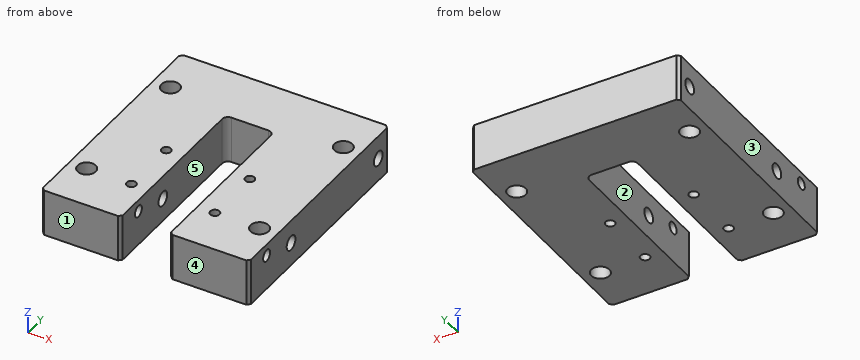
```python
from build123d import *

# Parameters (mm, degrees)
SKETCH_1_W          = 35.6
SKETCH_1_H          = 40
EXTRUDE_1_DEPTH     = 8
SKETCH_5_R          = 1
CUT_EXTRUDE_1_DEPTH = 42
SKETCH_6_W          = 8.3
SKETCH_6_H          = 60
CUT_EXTRUDE_2_DEPTH = 10
SKETCH_2_R          = 1.55
CUT_EXTRUDE_3_DEPTH = 10
HOLE_WIZARD_M2_1_D  = 1.6
HOLE_WIZARD_M3_2_D  = 2.5
FILLET_1_R          = 1
CHAMFER_1_SIZE      = 0.5


with BuildPart() as part:
    # 草图1 → 凸台-拉伸1 (new body)
    with BuildSketch(Plane.XY):
        Rectangle(SKETCH_1_W, SKETCH_1_H)
    extrude(amount=EXTRUDE_1_DEPTH)

    # 草图5 → 切除-拉伸1 (cut)
    with BuildSketch(Plane.ZY.offset(17.8)):
        with Locations((6, -15)):
            Circle(SKETCH_5_R)
    extrude(amount=-CUT_EXTRUDE_1_DEPTH, mode=Mode.SUBTRACT)

    # 草图6 → 切除-拉伸2 (cut)
    with BuildSketch(Plane.XY.offset(8)):
        with Locations((0, -20)):
            Rectangle(SKETCH_6_W, SKETCH_6_H)
    extrude(amount=-CUT_EXTRUDE_2_DEPTH, mode=Mode.SUBTRACT)

    # 草图2 → 切除-拉伸3 (cut)
    with BuildSketch(Plane.XY.offset(8)):
        with Locations((14.8, 12)):
            Circle(SKETCH_2_R)
        with Locations((-14.8, 12)):
            Circle(SKETCH_2_R)
        with Locations((-14.8, -12)):
            Circle(SKETCH_2_R)
        with Locations((14.8, -12)):
            Circle(SKETCH_2_R)
    extrude(amount=-CUT_EXTRUDE_3_DEPTH, mode=Mode.SUBTRACT)

    # M2 螺纹孔1 (through all)
    with Locations(Plane.XY.offset(8)):
        with Locations((-7.15, -12), (-7.15, -2)):
            hole_wizard_m2_1 = Hole(HOLE_WIZARD_M2_1_D / 2)

    # 镜向1: M2 螺纹孔1 across plane
    add(hole_wizard_m2_1.mirror(Plane(origin=(0, 0, 0), x_dir=(0, 0, 1), z_dir=(1, 0, 0))), mode=Mode.SUBTRACT)

    # M3 螺纹孔2 (through all)
    with Locations(Plane.ZY.offset(17.8)):
        with Locations((4, 17), (4, -8)):
            Hole(HOLE_WIZARD_M3_2_D / 2)

    # 圆角1
    fillet_1_edges = [part.edges().sort_by_distance(p)[0] for p in [
        (4.15, 10, 4),
        (-4.15, 10, 4),
    ]]
    fillet(fillet_1_edges, radius=FILLET_1_R)

    # 倒角1
    chamfer_1_edges = [part.edges().sort_by_distance(p)[0] for p in [
        (4.15, -20, 4),
        (-4.15, -20, 4),
        (17.8, -20, 4),
        (-17.8, -20, 4),
        (-17.8, 20, 4),
        (17.8, 20, 4),
    ]]
    chamfer(chamfer_1_edges, length=CHAMFER_1_SIZE)


solid = part.part
```
Model file for the job. Use its own axes, mm. Face numbers are marked on the shaded views. A direction names the side the tool comes from. Coordinates: 2 decimals unless noted, no trailing zeros. Order: outer loops, then holes, each group sorted by start corner. A loop starts at its lowest first (then second) coordinate and runs counter-clockwise, first axis right, second up. Notation, with made-up numbers: (66.5, 62.5) -> (110.5, 62.5) arc R20 ccw to (110.5, 98.5) -> close; hole circle Ø10 at (-7.75, -20). An arc over 180 degrees is marked (long way). Return JSON: item names as keys, results as strings.
Item 1: 3-axis set-ups, long thin cutter, end or side, ignore diameter. For the marked faces 1 and 2: which of +Z, -Z, +X, -X, +Y, -Y reach the whole face in a straight line?
Model answer:
{"face 1": "+Z, -Z, +X, -X, -Y", "face 2": "+Z, -Z, -Y"}
Item 2: Wall check: line 1 along Y through (x, z) = (9.25, 4); line 2 along Y through (x, z) = (7.15, 6); line 3 along Y through (x, z) = (11.5, 6). Give the ranges that are in metal, low to high. Write a range as from..to.
Model answer:
{"line 1": "y = -20..-9.25, -6.75..15.75, 18.25..20", "line 2": "y = -20..-16, -14..-12.8, -11.2..-2.8, -1.2..20", "line 3": "y = -20..-16, -14..20"}
Item 3: Slice it at C-C (y = 8). Write the cut outline in (x, z), then the cut area to 3 significant figures.
Model answer:
{"outline": "(-17.8, 0) -> (-4.15, 0) -> (-4.15, 8) -> (-17.8, 8) -> close; (4.15, 0) -> (17.8, 0) -> (17.8, 8) -> (4.15, 8) -> close", "area": "218 mm²"}
Item 4: Pin check, flat tips, straight feed: P1, Ø1.2, axis at y = -15, z = 6, coming from the -X side; P2, Ø4, axis at x = -0.5, z = 6, coming from the -Y side. Stop position of each tip, or through.
Model answer:
{"P1": "passes through", "P2": "stops at y = 10"}
Item 5: Slice it at B-B (z = 6). Count the separate pieces of the cut face and the enclosed holes in it, then the cut area to 3 significant figures.
Model answer:
{"separate pieces": "3", "enclosed holes": "8", "area": "1,080 mm²"}
Item 6: Slice it at A-A (x = 7.15). Write the cut outline in (y, z), then the cut area to 3 significant figures.
Model answer:
{"outline": "(-20, 0) -> (-12.8, 0) -> (-12.8, 8) -> (-20, 8) -> close; (-11.2, 0) -> (-2.8, 0) -> (-2.8, 8) -> (-11.2, 8) -> close; (-1.2, 0) -> (20, 0) -> (20, 8) -> (-1.2, 8) -> close; hole circle Ø2 at (-15, 6); hole circle Ø2.5 at (-8, 4); hole circle Ø2.5 at (17, 4)", "area": "281 mm²"}
Item 7: Mould opens along X. For the marked faces 3, 4 and 5 say: pulls with the +X half, pulls with the -X half, needs draft (parallel to the pull), parting line crosses it, or undercut.
Model answer:
{"face 3": "pulls with the -X half", "face 4": "needs draft", "face 5": "undercut"}
Item 8: Slice it at D-D (y = -12). Write the cut outline in (x, z), then the cut area to 3 significant figures.
Model answer:
{"outline": "(-17.8, 0) -> (-16.35, 0) -> (-16.35, 8) -> (-17.8, 8) -> close; (-13.25, 0) -> (-7.95, 0) -> (-7.95, 8) -> (-13.25, 8) -> close; (-6.35, 0) -> (-4.15, 0) -> (-4.15, 8) -> (-6.35, 8) -> close; (4.15, 0) -> (6.35, 0) -> (6.35, 8) -> (4.15, 8) -> close; (7.95, 0) -> (13.25, 0) -> (13.25, 8) -> (7.95, 8) -> close; (16.35, 0) -> (17.8, 0) -> (17.8, 8) -> (16.35, 8) -> close", "area": "143 mm²"}
